```python
from build123d import *

# Parameters (mm, degrees)
SKETCH_1_R          = 12.2
EXTRUDE_1_DEPTH     = 30.8
SKETCH_2_R          = 3.2
EXTRUDE_2_DEPTH     = 1.8
SKETCH_3_R          = 1
EXTRUDE_3_DEPTH     = 6.5
SKETCH_4_R          = 1.5
CUT_EXTRUDE_1_DEPTH = 2
EXTRUDE_START       = 1.6
SKETCH_5_R          = 3.2
SKETCH_5_W          = 2
SKETCH_5_H          = 0.3
EXTRUDE_4_DEPTH     = 1.6
SKETCH_6_W          = 2
SKETCH_6_H          = 0.3
EXTRUDE_5_DEPTH     = 2.4
SKETCH_7_R          = 1
CUT_EXTRUDE_2_DEPTH = 2
SKETCH_8_R          = 0.5
CUT_EXTRUDE_4_DEPTH = 0.3
FILLET_4_R          = 0.4


with BuildPart() as part:
    # 草图1 → 凸台-拉伸1 (new body)
    with BuildSketch(Plane(origin=(0, 0, 0), x_dir=(1, 0, 0), z_dir=(0, 1, 0))):
        with Locations(Location((0, 0, 0), (0, 0, 90))):
            Circle(SKETCH_1_R)
    extrude(amount=EXTRUDE_1_DEPTH)

    # 草图2 → 凸台-拉伸2 (add)
    with BuildSketch(Plane(origin=(0, 30.8, 0), x_dir=(1, 0, 0), z_dir=(0, 1, 0))):
        with Locations(Location((0, 0, 0), (0, 0, 270))):
            Circle(SKETCH_2_R)
    extrude(amount=EXTRUDE_2_DEPTH)

    # 草图3 → 凸台-拉伸3 (add)
    with BuildSketch(Plane(origin=(0, 32.6, 0), x_dir=(1, 0, 0), z_dir=(0, 1, 0))):
        with Locations(Location((0, 0, 0), (0, 0, 90))):
            Circle(SKETCH_3_R)
    extrude(amount=EXTRUDE_3_DEPTH)

    # 草图4 → 切除-拉伸1 (cut)
    with BuildSketch(Plane(origin=(0, 30.8, 0), x_dir=(1, 0, 0), z_dir=(0, 1, 0))):
        with Locations(Location((7.70361619, -3.592255225, 0), (0, 0, 270))):
            Circle(SKETCH_4_R)
        with Locations(Location((-7.70361619, 3.592255225, 0), (0, 0, 270))):
            Circle(SKETCH_4_R)
    extrude(amount=-CUT_EXTRUDE_1_DEPTH, mode=Mode.SUBTRACT)

    # 草图5 → 凸台-拉伸4 (add)
    with BuildSketch(Plane.XZ.offset(EXTRUDE_START)):
        with Locations(Location((0, 0, 0), (0, 0, 90))):
            Circle(SKETCH_5_R)
        with Locations((-9, 0)):
            Rectangle(SKETCH_5_W, SKETCH_5_H)
        with Locations((9, 0)):
            Rectangle(SKETCH_5_W, SKETCH_5_H)
    extrude(amount=-EXTRUDE_4_DEPTH)

    # 草图6 → 凸台-拉伸5 (add)
    with BuildSketch(Plane.XZ.offset(1.6)):
        with Locations((-9, 0)):
            Rectangle(SKETCH_6_W, SKETCH_6_H)
        with Locations((9, 0)):
            Rectangle(SKETCH_6_W, SKETCH_6_H)
    extrude(amount=EXTRUDE_5_DEPTH)

    # 草图7 → 切除-拉伸2 (cut)
    with BuildSketch(Plane.XZ.offset(1.6)):
        with Locations(Location((0, 0, 0), (0, 0, 270))):
            Circle(SKETCH_7_R)
    extrude(amount=-CUT_EXTRUDE_2_DEPTH, mode=Mode.SUBTRACT)

    # 草图8 → 切除-拉伸4 (cut)
    with BuildSketch(Plane(origin=(0, 0, -0.15), x_dir=(-1, 0, 0), z_dir=(0, 0, -1))):
        with Locations((9, -2.5)):
            Circle(SKETCH_8_R)
        with Locations(Location((-9, -2.5, 0), (0, 0, 180))):
            Circle(SKETCH_8_R)
    extrude(amount=-CUT_EXTRUDE_4_DEPTH, mode=Mode.SUBTRACT)

    # 圆角4
    fillet_4_edges = [part.edges().sort_by_distance(p)[0] for p in [
        (-10, -4, 0),
        (-8, -4, 0),
        (10, -4, 0),
        (8, -4, 0),
    ]]
    fillet(fillet_4_edges, radius=FILLET_4_R)


solid = part.part
```
Could you check a few things on this model? Use its own coordinates, in mm. A direction names the side the tool comes from. Round coordinates to 2 decimals unless told otherwise and drop trailing zeros. Order: outer loops, then holes, each group sorted by start corner. A loop starts at its lowest first (then second) coordinate and runs counter-clockwise, first axis right, second up. Notation, with made-up numbers: M -31,-15 L -27,-15 A18 cw -27,11 Z; hole C 89,2.5 d6. An arc over 180 degrees is marked long. One line per question, with ' | ' between items. Start each with the question number.
(1) Suppose I cut it at C-C on z = 4. List the corners of the cut face in (x, y) for me, then the cut area to 3 significant figures.
(2) For faces 1 (the face through (-6.439, 29.814, -2.786)), 2 (the face through (-9, -1.5, 0.15)), 3 (the face through (-9, -1.5, -0.15)), 4 (the face through (1.947, -0.811, -2.539)), which set-ups out of +Z, -Z, +X, -X, +Y, -Y let a thin tool reach every point of the face, with its end or its side?
(3) Thinking about a two-plate mould opening in Z: for faces 5 (the face through (9, -1.6, 0.15)), 6 (the face through (8, 28.8, 4)), 7 (the face through (-1.947, 31.687, -2.539)), which applies, +Z half, -Z half, draft (parallel to the pull), parting line (faces both ways), or undercut?
(4) For P1, Ø2.5, axis at x = 7.7, z = 3.59, coming from the +Y side; P2, Ø2, axis at y = 16.5, z = 8.5, coming from the -X side; P3, Ø1, axis at x = -7, z = 4.5, coming from the -Y side, each with a flat end and sliding along its axis, tell me the tip position at first contact or that it passes through.
(5) Suppose I cut it at A-A on y = -2.5. List the corners of the cut face in (x, z) for me, then the cut area to 3 significant figures.
(6) Suppose I cut it at D-D on y = 25. List the corners of the cut face in (x, z) for me.
(7) Suppose I cut it at B-B on x = 0. List the corners of the cut face in (y, z) for me.
(8) Please list where these lines run through material, in increasing order: line 1 along Y through (x, z) = (9, 0); line 2 along Y through (x, z) = (0.75, 1.5); line 3 along Y through (x, z) = (-3, 6.5).
Geometry results:
1) outline: M -11.53,0 L 11.53,0 L 11.53,30.8 L 9.15,30.8 L 9.15,28.8 L 6.26,28.8 L 6.26,30.8 L -11.53,30.8 Z | area: 704 mm²
2) face 1: +Y | face 2: +Z, -X, -Y | face 3: -Z, -X, -Y | face 4: -Y
3) face 5: +Z half | face 6: undercut | face 7: parting line
4) P1: y = 28.8 | P2: x = -9.62 | P3: y = 0
5) outline: M -10,-0.15 L -9.5,-0.15 L -9.5,0.15 L -10,0.15 Z; M -8.5,-0.15 L -8,-0.15 L -8,0.15 L -8.5,0.15 Z; M 8,-0.15 L 8.5,-0.15 L 8.5,0.15 L 8,0.15 Z; M 9.5,-0.15 L 10,-0.15 L 10,0.15 L 9.5,0.15 Z | area: 0.600 mm²
6) outline: C 0,0 d24.4
7) outline: M -1.6,-3.2 L 0,-3.2 L 0,-12.2 L 30.8,-12.2 L 30.8,-3.2 L 32.6,-3.2 L 32.6,-1 L 39.1,-1 L 39.1,1 L 32.6,1 L 32.6,3.2 L 30.8,3.2 L 30.8,12.2 L 0,12.2 L 0,3.2 L -1.6,3.2 L -1.6,1 L 0.4,1 L 0.4,-1 L -1.6,-1 Z
8) line 1: -4 to -3, -2 to 30.8 | line 2: -1.6 to 32.6 | line 3: 0 to 30.8
